Check sheet for the modelled part. Datum: model origin and axes. Units: mm. Face numbers are marked on the shaded views. A direction names the side the tool comes from. Coordinates: 2 decimals unless noted, no trailing zeros. Loops run counter-clockwise (first coordinate to the right, second up) from the corner with the lowest first, then second, coordinate; pieces in that order, holes last.
```python
from build123d import *

# Parameters (mm, degrees)
BOSS_EXTRUDE1_DEPTH = 3
BOSS_EXTRUDE2_DEPTH = 3
SKETCH3_R           = 2.5
BOSS_EXTRUDE3_DEPTH = 1.5
CHAMFER1_SIZE       = 0.5


with BuildPart() as part:
    # Sketch1 → Boss-Extrude1 (new body)
    with BuildSketch(Plane.XY):
        with BuildLine():
            Line((1, 0), (17, 0))
            ThreePointArc((17, 0), (17.707106781, 0.292893219), (18, 1))
            Line((18, 1), (18, 23))
            ThreePointArc((18, 23), (17.707106781, 23.707106781), (17, 24))
            Line((17, 24), (1, 24))
            ThreePointArc((1, 24), (0.292893219, 23.707106781), (0, 23))
            Line((0, 23), (0, 1))
            ThreePointArc((0, 1), (0.292893219, 0.292893219), (1, 0))
        make_face()
    extrude(amount=BOSS_EXTRUDE1_DEPTH)

    # Sketch2 → Boss-Extrude2 (add)
    with BuildSketch(Plane.XY.offset(3)):
        with BuildLine():
            Line((1, 0), (17, 0))
            ThreePointArc((17, 0), (17.707106781, 0.292893219), (18, 1))
            Line((18, 1), (18, 4))
            Line((18, 4), (0, 4))
            Line((0, 4), (0, 1))
            ThreePointArc((0, 1), (0.292893219, 0.292893219), (1, 0))
        make_face()
    extrude(amount=BOSS_EXTRUDE2_DEPTH)

    # Sketch3 → Boss-Extrude3 (add)
    with BuildSketch(Plane(origin=(0, 0, 0), x_dir=(-1, 0, 0), z_dir=(0, 0, -1))):
        with Locations((-15, 21)):
            Circle(SKETCH3_R)
        with Locations((-3, 7)):
            Circle(SKETCH3_R)
    extrude(amount=BOSS_EXTRUDE3_DEPTH)

    # Chamfer1
    chamfer1_edges = [part.edges().sort_by_distance(p)[0] for p in [
        (17.5, 21, -1.5),
        (5.5, 7, -1.5),
    ]]
    chamfer(chamfer1_edges, length=CHAMFER1_SIZE)


solid = part.part
```
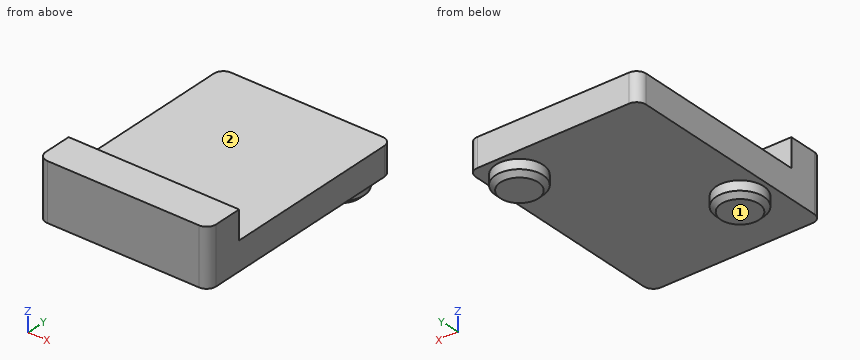
1) Set-up check for the marked faces 1 and 2: record each of +Z, -Z, +X, -X, +Y, -Y from which the full face is reachable in a straight line by a thin tool's end or side.
Answer sheet:
face 1: -Z, +X, -X, +Y, -Y
face 2: +Z, +X, -X, +Y
2) Section check B-B on y = 21. Enter the section's corners in (x, z), plus the area to 4 significant figures.
Answer sheet:
outline: (0, 0) - (12.5, 0) - (12.5, -1) - (13, -1.5) - (17, -1.5) - (17.5, -1) - (17.5, 0) - (18, 0) - (18, 3) - (0, 3) - close
area: 61.25 mm2
3) Section check C-C on z = 4.5. Enter the section's corners in (x, y), plus the area to 3 significant figures.
Answer sheet:
outline: (0, 1) arc R1 ccw to (1, 0) - (17, 0) arc R1 ccw to (18, 1) - (18, 4) - (0, 4) - close
area: 71.6 mm2
4) Depth check by flat-ended pin: pin 1 (3 mm diameter, centred on y = 9, z = 0, fed in from -X); pin 2 (2 mm diameter, centred on x = 10.5, y = 16, fed in from -Z); pin 3 (1 mm diameter, centred on x = 15, y = 15, fed in from +Z); pin 4 (1.5 mm diameter, centred on x = 10.5, z = 5, fed in from +Y). Enter the tip coordinate at first touch or a pass-through.
Answer sheet:
pin 1: stops at x = 0
pin 2: stops at z = 0
pin 3: stops at z = 3
pin 4: stops at y = 4
5) Scan lines: line 1 (Z direction, x = 11, y = 22); line 2 (Y direction, x = 12.5, z = 3.5); line 3 (Z direction, x = 1.5, y = 2). Record each from-to range of solid material in increasing order.
Answer sheet:
line 1: z = 0 to 3
line 2: y = 0 to 4
line 3: z = 0 to 6
6) Section check D-D on x = 3. Enter the section's corners in (y, z), plus the area to 4 significant figures.
Answer sheet:
outline: (0, 0) - (4.5, 0) - (4.5, -1) - (5, -1.5) - (9, -1.5) - (9.5, -1) - (9.5, 0) - (24, 0) - (24, 3) - (4, 3) - (4, 6) - (0, 6) - close
area: 91.25 mm2
7) Section check A-A on x = 10. Enter the section's corners in (y, z), plus the area to 3 significant figures.
Answer sheet:
outline: (0, 0) - (24, 0) - (24, 3) - (4, 3) - (4, 6) - (0, 6) - close
area: 84.0 mm2
